Work out the finished part from the listing and answer in its coordinate system (mm). Round coordinates to 2 decimals unless told otherwise and drop trailing zeros. Order: outer loops, then holes, each group sorted by start corner. A loop starts at its lowest first (then second) coordinate and runs counter-clockwise, first axis right, second up. Notation, with made-up numbers: M -30,21.25 L 12,21.25 A30 cw 12,48.25 Z; hole C 14,-23 d2. An arc over 180 degrees is marked long. Return JSON: item names as keys, results as strings.
from build123d import *

# Parameters (mm, degrees)
BOSS_EXTRUDE1_DEPTH     = 6.35
F_1_4_CLEARANCE_HOLE1_D = 6.7564
CUT_EXTRUDE1_DEPTH      = 376.065853402
FILLET1_R               = 2.54


with BuildPart() as part:
    # Sketch1 → Boss-Extrude1 (new body)
    with BuildSketch(Plane(origin=(0, 0, 0), x_dir=(1, 0, 0), z_dir=(0, 1, 0))):
        Polygon((-177.8, 307.958633586), (-22.225, 38.494829198), (22.225, 38.494829198), (177.8, 307.958633586), (139.305170802, 330.183633586), (-139.305170802, 330.183633586), align=None)
    extrude(amount=BOSS_EXTRUDE1_DEPTH)

    # 1/4 Clearance Hole1 (through all)
    with Locations(Plane(origin=(0, 6.35, 0), x_dir=(1, 0, 0), z_dir=(0, 1, 0))):
        with Locations((0, 299.260881198), (0, 70.660881198), (0, 184.960881198)):
            Hole(F_1_4_CLEARANCE_HOLE1_D / 2)

    # Sketch6 → Cut-Extrude1 (cut, through all)
    with BuildSketch(Plane(origin=(0, 6.35, 0), x_dir=(1, 0, 0), z_dir=(0, 1, 0))):
        with BuildLine():
            Line((-146.190878382, 304.41642896), (-143.219078382, 299.269120371))
            ThreePointArc((-143.219078382, 299.269120371), (-144.455585401, 294.654413351), (-149.07029242, 295.890920371))
            Line((-149.07029242, 295.890920371), (-152.04209242, 301.03822896))
            ThreePointArc((-152.04209242, 301.03822896), (-150.805585401, 305.65293598), (-146.190878382, 304.41642896))
        make_face()
        with BuildLine():
            Line((-85.57029242, 185.90569409), (-88.54209242, 191.05300268))
            ThreePointArc((-88.54209242, 191.05300268), (-87.305585401, 195.667709699), (-82.690878382, 194.43120268))
            Line((-82.690878382, 194.43120268), (-79.719078382, 189.28389409))
            ThreePointArc((-79.719078382, 189.28389409), (-80.955585401, 184.669187071), (-85.57029242, 185.90569409))
        make_face()
        with BuildLine():
            Line((146.190878382, 304.41642896), (143.219078382, 299.269120371))
            ThreePointArc((143.219078382, 299.269120371), (144.455585401, 294.654413351), (149.07029242, 295.890920371))
            Line((149.07029242, 295.890920371), (152.04209242, 301.03822896))
            ThreePointArc((152.04209242, 301.03822896), (150.805585401, 305.65293598), (146.190878382, 304.41642896))
        make_face()
        with BuildLine():
            Line((85.57029242, 185.90569409), (88.54209242, 191.05300268))
            ThreePointArc((88.54209242, 191.05300268), (87.305585401, 195.667709699), (82.690878382, 194.43120268))
            Line((82.690878382, 194.43120268), (79.719078382, 189.28389409))
            ThreePointArc((79.719078382, 189.28389409), (80.955585401, 184.669187071), (85.57029242, 185.90569409))
        make_face()
    extrude(amount=-CUT_EXTRUDE1_DEPTH, mode=Mode.SUBTRACT)

    # Fillet1
    fillet1_edges = [part.edges().sort_by_distance(p)[0] for p in [
        (22.225, 3.175, -38.494829198),
        (-22.225, 3.175, -38.494829198),
        (-177.8, 3.175, -307.958633586),
        (-139.305170802, 3.175, -330.183633586),
        (139.305170802, 3.175, -330.183633586),
        (177.8, 3.175, -307.958633586),
    ]]
    fillet(fillet1_edges, radius=FILLET1_R)


solid = part.part
Item 1: Consider line 1 along Z through (x, y) = (0, 4.5); line 2 along X through (y, z) = (4.5, -187); line 3 along Z through (x, y) = (-84, 4). Determine where each line is inside the solid, lowest interval first. Write a range as [from, to].
Output:
{"line 1": "z = [-330.18, -302.64], [-295.88, -188.34], [-181.58, -74.04], [-67.28, -38.49]", "line 2": "x = [-107.96, -86.2], [-79.32, -2.69], [2.69, 79.32], [86.2, 107.96]", "line 3": "z = [-330.18, -195.71], [-184.5, -145.49]"}
Item 2: This flat-tipped pin is pushed along its axis until it touches: pin 1 (1.5 mm diameter, centred on y = 2.5, z = -189.5, fed in from -X). Where does it stop, or does it pass through?
Output:
{"pin 1": "stops at x = -109.84"}
Item 3: Find section A-A (y = 2). State how many separate pieces and enclosed holes the cut face has, plus the area to 3 significant figures.
Output:
{"separate pieces": "1", "enclosed holes": "7", "area": "60,500 mm^2"}
Item 4: Find section B-B (x = 41.5). Determine the outline of the cut face in (y, z), plus the area to 3 significant figures.
Output:
{"outline": "M 0,-330.18 L 6.35,-330.18 L 6.35,-71.88 L 0,-71.88 Z", "area": "1,640 mm^2"}
Item 5: Find section C-C (z = -241). Determine the outline of the cut face in (x, y).
Output:
{"outline": "M -139.14,0 L 139.14,0 L 139.14,6.35 L -139.14,6.35 Z"}
